from build123d import *

# Parameters (mm, degrees)
F1_DEPTH = 600
F2_W     = 52.7
F2_H     = 25.4
F3_DEPTH = 5
F4_W     = 6.35
F4_H     = 10
F5_DEPTH = 5


with BuildPart() as f1:
    # F0 (on Front) → F1 (new body)
    with BuildSketch(Plane.XZ):
        with BuildLine():
            Line((-40, 0), (0, 0))
            Line((0, 0), (0, 5))
            Line((0, 5), (-10.75, 5))
            Line((-10.75, 5), (-10.75, 11.7))
            Line((-10.75, 11.7), (-12.478163, 11.7))
            Line((-12.478163, 11.7), (-16, 17.8))
            ThreePointArc((-16, 17.8), (-20, 33.236504), (-24, 17.8))
            Line((-24, 17.8), (-27.521837, 11.7))
            Line((-27.521837, 11.7), (-29.25, 11.7))
            Line((-29.25, 11.7), (-29.25, 5))
            Line((-29.25, 5), (-40, 5))
            Line((-40, 5), (-40, 0))
        make_face()
    extrude(amount=F1_DEPTH)

    # F2 (on face) → F3 (join, through all)
    with BuildSketch(Plane.XY.offset(5)):
        with Locations((-20, -587.3)):
            Rectangle(F2_W, F2_H)
        with Locations((-20, -12.7)):
            Rectangle(F2_W, F2_H)
    extrude(amount=-F3_DEPTH)

    # F4 (on face) → F5 (join, through all)
    with BuildSketch(Plane.XY.offset(5)):
        with Locations((-43.175, -300)):
            Rectangle(F4_W, F4_H)
    extrude(amount=-F5_DEPTH)


solid = f1.part
Here's how the part is built. I have some questions about the finished solid (model axes, mm). A direction names the side the tool comes from. Coordinates: 2 decimals unless noted, no trailing zeros. Write each loop counter-clockwise with the first axis right and the second up, starting at its lowest first coordinate (ties: lowest second). Pieces come first, ordered by that corner, then holes.
1) If we section it at A-A (y = -274): List the corners of the cut face in (x, z) for me, plus the area to 3 significant figures.
Filled in:
outline: (-40, 0) - (0, 0) - (0, 5) - (-10.75, 5) - (-10.75, 11.7) - (-12.48, 11.7) - (-16, 17.8) arc R8.24 ccw (long way) to (-24, 17.8) - (-27.52, 11.7) - (-29.25, 11.7) - (-29.25, 5) - (-40, 5) - close
area: 602 mm2
2) If I drill on line 1 (Z direction, x = -35, y = -524); line 2 (X direction, y = -406, z = 4); line 3 (X direction, y = -185, z = 21.5), over which ranges is the centre line in solid material (lowest first)?
Filled in:
line 1: z = 0 to 5
line 2: x = -40 to 0
line 3: x = -27.46 to -12.54
3) Which directions (+Z, -Z, +X, -X, +Y, -Y) give clear straight access to the entire face, cutting with the end or side of a thin tool? Please do faces 1 (the face through (-36, -296, 5)), 2 (the face through (-6, -296, 5)), 3 (the face through (-20, -600, 12)).
Filled in:
face 1: +Z, -X, +Y, -Y
face 2: +Z, +X, +Y, -Y
face 3: +Z, -Z, +X, -X, -Y
4) I'm going to push flat-ended pins straight in: pin 1 (2 mm diameter, centred on y = -349.5, z = 9.5, fed in from -X); pin 2 (2 mm diameter, centred on y = -237.5, z = 7.5, fed in from +X); pin 3 (5 mm diameter, centred on x = -10, z = 18.5, fed in from +Y); pin 4 (4 mm diameter, centred on y = -194.5, z = 2.5, fed in from +X). Where does each tip first touch, or does it pass through?
Filled in:
pin 1: stops at x = -29.25
pin 2: stops at x = -10.75
pin 3: passes through
pin 4: stops at x = 0
5) If we section it at B-B (z = 25): List the corners of the cut face in (x, y) for me, plus the area to 3 significant figures.
Filled in:
outline: (-28.24, -600) - (-11.76, -600) - (-11.76, 0) - (-28.24, 0) - close
area: 9,880 mm2
